```python
from build123d import *

# Parameters (mm, degrees)
F0_W     = 60
F0_H     = 40
F1_DEPTH = 40
F2_T     = -5
F3_R     = 5


with BuildPart() as f1:
    # F0 (on Top) → F1 (new body)
    with BuildSketch(Plane.XY):
        Rectangle(F0_W, F0_H)
    extrude(amount=F1_DEPTH)

    # F2
    f2_openings = [f1.faces().sort_by_distance(p)[0] for p in [
        (0, 0, 40),
    ]]
    offset(amount=F2_T, openings=f2_openings)

    # F3
    f3_edges = [f1.edges().sort_by_distance(p)[0] for p in [
        (-30, 20, 20),
        (30, 20, 20),
        (-30, -20, 20),
        (30, -20, 20),
        (-25, -15, 22.5),
        (-25, 15, 22.5),
        (25, -15, 22.5),
        (25, 15, 22.5),
        (0, 20, 0),
        (0, -20, 0),
    ]]
    fillet(f3_edges, radius=F3_R)


solid = f1.part
```
Verification items for the finished model (mm, model axes). A direction names the side the tool comes from. Coordinates: 2 decimals unless noted, no trailing zeros. Loops run counter-clockwise (first coordinate to the right, second up) from the corner with the lowest first, then second, coordinate; pieces in that order, holes last. Notation, with made-up numbers: (41, 36.5) -> (53, 36.5) arc R6 ccw to (53, 44.5) -> close; hole circle Ø8 at (38, 39.5). An arc over 180 degrees is marked (long way). Put each result on its own line as item: value.
1. Section check C-C, the plane x = -6.5. Record the boundary of the cut face in (y, z), then the cut area to 3 significant figures.
Result set:
outline: (-20, 5) arc R5 ccw to (-15, 0) -> (15, 0) arc R5 ccw to (20, 5) -> (20, 40) -> (15, 40) -> (15, 5) -> (-15, 5) -> (-15, 40) -> (-20, 40) -> close
area: 539 mm^2
2. Gauge pin test, flat ends, axial feed: P1, Ø9, axis at x = -7.5, y = -5.5, coming from the +Z side; P2, Ø4, axis at x = -23.5, y = -15, coming from the -Z side. Record the tip position at first contact, or that the pin passes through.
Result set:
P1: stops at z = 5
P2: stops at z = 0
3. Section check A-A, the plane z = 24. Record the boundary of the cut face in (x, y), then the cut area to 3 significant figures.
Result set:
outline: (-30, -15) arc R5 ccw to (-25, -20) -> (25, -20) arc R5 ccw to (30, -15) -> (30, 15) arc R5 ccw to (25, 20) -> (-25, 20) arc R5 ccw to (-30, 15) -> close; hole (-25, -10) arc R5 ccw to (-20, -15) -> (20, -15) arc R5 ccw to (25, -10) -> (25, 10) arc R5 ccw to (20, 15) -> (-20, 15) arc R5 ccw to (-25, 10) -> close
area: 900 mm^2
4. Section check B-B, the plane y = -14. Record the boundary of the cut face in (x, z).
Result set:
outline: (-30, 0) -> (30, 0) -> (30, 40) -> (23, 40) -> (23, 5) -> (-23, 5) -> (-23, 40) -> (-30, 40) -> close
5. Section check D-D, the plane y = 2.5. Record the boundary of the cut face in (x, z).
Result set:
outline: (-30, 0) -> (30, 0) -> (30, 40) -> (25, 40) -> (25, 5) -> (-25, 5) -> (-25, 40) -> (-30, 40) -> close
6. Thickness scan on line 1 (Y direction, x = 5, z = 18.5); line 2 (X direction, y = 6, z = 6); line 3 (Z direction, x = -14.5, y = 8). Record the ranges inside material, lowest first.
Result set:
line 1: y = -20 to -15, 15 to 20
line 2: x = -30 to -25, 25 to 30
line 3: z = 0 to 5
7. Tool access check on faces 1 (the face through (25, 0, 22)), 2 (the face through (0, -20, 22)). Record the directions out of +Z, -Z, +X, -X, +Y, -Y that give a thin tool (end or side, any length) a straight path to the whole face; none if there is none.
Result set:
face 1: +Z
face 2: +Z, -Z, +X, -X, -Y
8. Mould release check, pull along Y, two halves, no side actions. Record for faces 3 (the face through (0, 15, 22)), 4 (the face through (0, -17, 40)), 5 (the face through (29, 18, 20)): pulls with the +Y half, pulls with the -Y half, needs draft (parallel to the pull), parting line crosses it, or undercut.
Result set:
face 3: undercut
face 4: needs draft
face 5: pulls with the +Y half
